Here's how the part is built. I have some questions about the finished solid (model axes, mm). Round coordinates to 2 decimals unless told otherwise and drop trailing zeros. Write each loop counter-clockwise with the first axis right and the second up, starting at its lowest first coordinate (ties: lowest second). Pieces come first, ordered by that corner, then holes. Notation, with made-up numbers: (67, 28) -> (116, 28) arc R20 ccw to (116, 62) -> close; hole circle Ø6 at (53, 53.5). An arc over 180 degrees is marked (long way). Put each result on its own line as item: value. Start each with the question number.
1) I want a section at C-C, the plane y = -997. List the corners of the cut face in (x, z) for me, then the cut area to 3 significant figures.
2) Will this pin go through, and if not, where does the flat tip stop? P1, Ø1, axis at y = -1417, z = 32.5, coming from the +X side.
3) I want a section at B-B, the plane x = 48. List the corners of the cut face in (y, z) for me.
4) We'd pull the mould along Z, two halves only. Please class faces 1 (the flat face through (38, -983, 31.75)), 2 (the flat face through (38, -983, 6.35)), 3 (the flat face through (38, -983, 0)), 4 (the flat face through (38, 0, 32)): released by +Z, released by -Z, zero draft, split by the parting line, or undercut.
5) If I drill on line 1 along Z through (x, y) = (61, -671); line 2 along Z through (x, y) = (65, -618.5); line 3 along X through (y, z) = (-392, 20), over which ranges is the centre line in solid material (lowest first)? Write a range as [from, to].
6) I want a section at A-A, the plane z = 19.5. List the corners of the cut face in (x, y) for me, then the cut area to 3 significant figures.
from build123d import *

# Parameters (mm, degrees)
F1_DEPTH = 1993.9


with BuildPart() as f1:
    # F0 (on Front) → F1 (new body)
    with BuildSketch(Plane.XZ):
        with BuildLine():
            ThreePointArc((0, 6.35), (1.859872, 1.859872), (6.35, 0))
            Line((6.35, 0), (69.85, 0))
            ThreePointArc((69.85, 0), (74.340128, 1.859872), (76.2, 6.35))
            Line((76.2, 6.35), (76.2, 31.75))
            ThreePointArc((76.2, 31.75), (74.340128, 36.240128), (69.85, 38.1))
            Line((69.85, 38.1), (6.35, 38.1))
            ThreePointArc((6.35, 38.1), (1.859872, 36.240128), (0, 31.75))
            Line((0, 31.75), (0, 6.35))
        make_face()
        with BuildLine():
            Line((63.5, 6.35), (12.7, 6.35))
            ThreePointArc((12.7, 6.35), (8.209872, 8.209872), (6.35, 12.7))
            Line((6.35, 12.7), (6.35, 25.4))
            ThreePointArc((6.35, 25.4), (8.209872, 29.890128), (12.7, 31.75))
            Line((12.7, 31.75), (63.5, 31.75))
            ThreePointArc((63.5, 31.75), (67.990128, 29.890128), (69.85, 25.4))
            Line((69.85, 25.4), (69.85, 12.7))
            ThreePointArc((69.85, 12.7), (67.990128, 8.209872), (63.5, 6.35))
        make_face(mode=Mode.SUBTRACT)
    extrude(amount=F1_DEPTH)


solid = f1.part
Findings:
1. outline: (0, 6.35) arc R6.35 ccw to (6.35, 0) -> (69.85, 0) arc R6.35 ccw to (76.2, 6.35) -> (76.2, 31.75) arc R6.35 ccw to (69.85, 38.1) -> (6.35, 38.1) arc R6.35 ccw to (0, 31.75) -> close; hole (6.35, 12.7) arc R6.35 ccw to (12.7, 6.35) -> (63.5, 6.35) arc R6.35 ccw to (69.85, 12.7) -> (69.85, 25.4) arc R6.35 ccw to (63.5, 31.75) -> (12.7, 31.75) arc R6.35 ccw to (6.35, 25.4) -> close
1. area: 1,290 mm2
2. P1: stops at x = 76.2
3. outline: (-1993.9, 0) -> (0, 0) -> (0, 6.35) -> (-1993.9, 6.35) -> close; (-1993.9, 31.75) -> (0, 31.75) -> (0, 38.1) -> (-1993.9, 38.1) -> close
4. face 1: undercut
4. face 2: undercut
4. face 3: released by -Z
4. face 4: zero draft
5. line 1: z = [0, 6.35], [31.75, 38.1]
5. line 2: z = [0, 6.53], [31.57, 38.1]
5. line 3: x = [0, 6.35], [69.85, 76.2]
6. outline: (0, -1993.9) -> (6.35, -1993.9) -> (6.35, 0) -> (0, 0) -> close; (69.85, -1993.9) -> (76.2, -1993.9) -> (76.2, 0) -> (69.85, 0) -> close
6. area: 25,300 mm2
